Check sheet for the modelled part. Datum: model origin and axes. Units: mm. A direction names the side the tool comes from. Round coordinates to 2 decimals unless told otherwise and drop trailing zeros. Write each loop counter-clockwise with the first axis right and the second up, starting at its lowest first coordinate (ties: lowest second). Pieces come first, ordered by that corner, then holes. Notation, with made-up numbers: M 31,-24.5 L 45,-24.5 A9 cw 45,-12.5 Z; hole C 4.5,-33.75 d2. An arc over 180 degrees is marked long. Put each result on its own line as item: value.
Autodesk Inventor part; units mm, degrees
ref_plane "to_bushings_XY" through (0, 0, 0) normal (0, 0, 1) x (1, 0, 0)
ref_plane "to_bushings_YZ" through (0, 0, 0) normal (1, 0, 0) x (0, 1, 0)
ref_plane "to_bushings_ZX" through (0, 0, 0) normal (0, 1, 0) x (0, 0, 1)
sketch "Sketch_8" plane through (0, 0, 0) normal (1, 0, 0) x (0, 0, -1)
  line L0 (-34, 18) -> (-34, -12)
  line L1 (-34, -12) -> (-33, -13)
  line L2 (-33, -13) -> (33, -13)
  line L3 (33, -13) -> (34, -12)
  line L4 (34, -12) -> (34, 18)
  line L5 (34, 18) -> (33, 19)
  line L6 (33, 19) -> (-33, 19)
  line L7 (-33, 19) -> (-34, 18)
extrude "Extrusion1" add sketch "Sketch_8" along normal mid plane 26
sketch "_____1" plane through (0, 0, 0) normal (0, 0, 1) x (1, 0, 0)
  line L0 (-14, -14) -> (14, -14)
  line L1 (14, -14) -> (14, 20)
  line L2 (14, 20) -> (-14, 20)
  line L3 (-14, 20) -> (-14, -14)
  line L4 (-13, 18) -> (-13, -12)
  line L5 (-13, -12) -> (-12, -13)
  line L6 (-12, -13) -> (12, -13)
  line L7 (12, -13) -> (13, -12)
  line L8 (13, -12) -> (13, 18)
  line L9 (13, 18) -> (12, 19)
  line L10 (12, 19) -> (-12, 19)
  line L11 (-12, 19) -> (-13, 18)
extrude "Extrusion2" cut sketch "_____1" along normal mid plane 68
sketch "_____2" plane through (0, 0, 0) normal (0, 1, 0) x (1, 0, 0)
  line L0 (-14, -35) -> (14, -35)
  line L1 (14, -35) -> (14, 35)
  line L2 (14, 35) -> (-14, 35)
  line L3 (-14, 35) -> (-14, -35)
  line L4 (-13, 33) -> (-13, -33)
  line L5 (-13, -33) -> (-12, -34)
  line L6 (-12, -34) -> (12, -34)
  line L7 (12, -34) -> (13, -33)
  line L8 (13, -33) -> (13, 33)
  line L9 (13, 33) -> (12, 34)
  line L10 (12, 34) -> (-12, 34)
  line L11 (-12, 34) -> (-13, 33)
extrude "Extrusion3" cut sketch "_____2" along normal mid plane 64
sketch "Sketch_1" plane through (0, 0, 0) normal (1, 0, 0) x (0, 0, -1)
  line L0 (34, 0) -> (-34, 0)
  line L1 (-34, 0) -> (-34, 10.3)
  line L2 (-34, 10.3) -> (-33.2, 9.5)
  line L3 (-33.2, 9.5) -> (-30, 9.5)
  line L4 (-30, 9.5) -> (-30, 10)
  line L5 (-30, 10) -> (-28.85, 10)
  line L6 (-28.85, 10) -> (-28.85, 9.5)
  line L7 (-28.85, 9.5) -> (28.85, 9.5)
  line L8 (28.85, 9.5) -> (28.85, 10)
  line L9 (28.85, 10) -> (30, 10)
  line L10 (30, 10) -> (30, 9.5)
  line L11 (30, 9.5) -> (33.2, 9.5)
  line L12 (33.2, 9.5) -> (34, 10.3)
  line L13 (34, 10.3) -> (34, 0)
  line L14 (34, 0) -> (-34, 0)
revolve "Revolution1" cut sketch "Sketch_1" angle 360 about axis through (0, 0, -34) along (0, 0, -1)
sketch "Sketch5" plane through (-12, 19, -33) normal (0, 1, 0) x (1, 0, 0)
  point P0 (12, -15)
hole "Hole1" at (0, 19, -18) direction (0, -1, 0) diameter 4.917 depth 19 countersink diameter 6 countersink angle 90
pattern_linear "Rectangular Pattern1" count 2 spacing 36 along (0, 0, 1) of "Hole1"
sketch "Sketch_3" plane through (0, 13, 0) normal (0, 1, 0) x (1, 0, 0)
  line L0 (13, 25) -> (-13, 25)
  line L1 (-13, 25) -> (-13, 27.5)
  line L2 (-13, 27.5) -> (-12.567, 27.067)
  line L3 (-12.567, 27.067) -> (6.567, 27.067)
  line L4 (6.567, 27.067) -> (7, 27.5)
  line L5 (7, 27.5) -> (7, 29)
  line L6 (7, 29) -> (13, 29)
  line L7 (13, 29) -> (13, 25)
  line L8 (13, 25) -> (-13, 25)
revolve "Revolution2" cut sketch "Sketch_3" angle 360 about axis through (13, 13, -25) along (1, 0, 0)
thread "Thread1"
pattern_linear "Rectangular Pattern2" count 2 spacing 50 along (0, 0, 1) of "Revolution2"
ref_plane "to_bushings_XY" through (0, 0, 0) normal (0, 0, 1) x (1, 0, 0)
ref_plane "to_bushings_YZ" through (0, 0, 0) normal (1, 0, 0) x (0, 1, 0)
ref_plane "to_bushings_ZX" through (0, 0, 0) normal (0, 1, 0) x (0, 0, 1)
ref_plane "to_rring_l_XY" through (0, 0, 28.85) normal (0, 0, -1) x (1, 0, 0)
ref_plane "to_rring_l_YZ" through (0, 0, 28.85) normal (1, 0, 0) x (0, -1, 0)
ref_plane "to_rring_l_ZX" through (0, 0, 28.85) normal (0, -1, 0) x (0, 0, -1)
ref_plane "to_rring_r_XY" through (0, 0, -28.85) normal (0, 0, 1) x (-1, 0, 0)
ref_plane "to_rring_r_YZ" through (0, 0, -28.85) normal (-1, 0, 0) x (0, -1, 0)
ref_plane "to_rring_r_ZX" through (0, 0, -28.85) normal (0, -1, 0) x (0, 0, 1)
properties part number "SLHSSW10_b"
1. Cross-section at B-B (z = -25). Enter the section's corners in (x, y).
Computed values:
outline: M -13,-12 L -12,-13 L 12,-13 L 13,-12 L 13,9 L 7,9 L 7,10.5 L 6.57,10.93 L -12.57,10.93 L -13,10.5 Z; M -13,15.5 L -12.57,15.07 L 6.57,15.07 L 7,15.5 L 7,17 L 13,17 L 13,18 L 12,19 L -12,19 L -13,18 Z; hole C 0,0 d19
2. Cross-section at D-D (z = -12.5). Enter the section's corners in (x, y).
Computed values:
outline: M -13,-12 L -12,-13 L 12,-13 L 13,-12 L 13,18 L 12,19 L -12,19 L -13,18 Z; hole C 0,0 d19
3. Access from +Z, -Z, +X, -X, +Y, -Y to the whole of each face (thin tool, end or side, straight path). Record for faces 4 (the flat face through (7, 15, 23)), 5 (the flat face through (-6, 9, -34)), 6 (the flat face through (-4, 9, 28.85)).
Computed values:
face 4: +X
face 5: -Z, +X, -X, +Y, -Y
face 6: none
4. Scan lines: probe 1 along X at (y, z) = (13, -18); probe 2 along Z at (x, y) = (1, 10); probe 3 along X at (y, z) = (0, 29.5). Record each from-to range of solid material in increasing order.
Computed values:
probe 1: x = -13 to -2.46, 2.46 to 13
probe 2: z = -33.75 to -20.25, -15.75 to 15.75, 20.25 to 33.75
probe 3: x = -13 to -10, 10 to 13
5. Release check for a two-part mould opening along X. For faces 1 (the cylindrical face through (-8.43, 4.38, -31.62)), 2 (the flat face through (0, 19, 0)), 3 (the flat face through (13, 3, 0)) record: +X half, -X half, draft (parallel to the pull), parting line (faces both ways), or undercut.
Computed values:
face 1: undercut
face 2: draft
face 3: +X half
6. Cross-section at A-A (y = 13). Count the separate pieces of the cut face and the enclosed holes in it, then the cut area to 3 significant figures.
Computed values:
separate pieces: 3
enclosed holes: 2
area: 1,470 mm2
